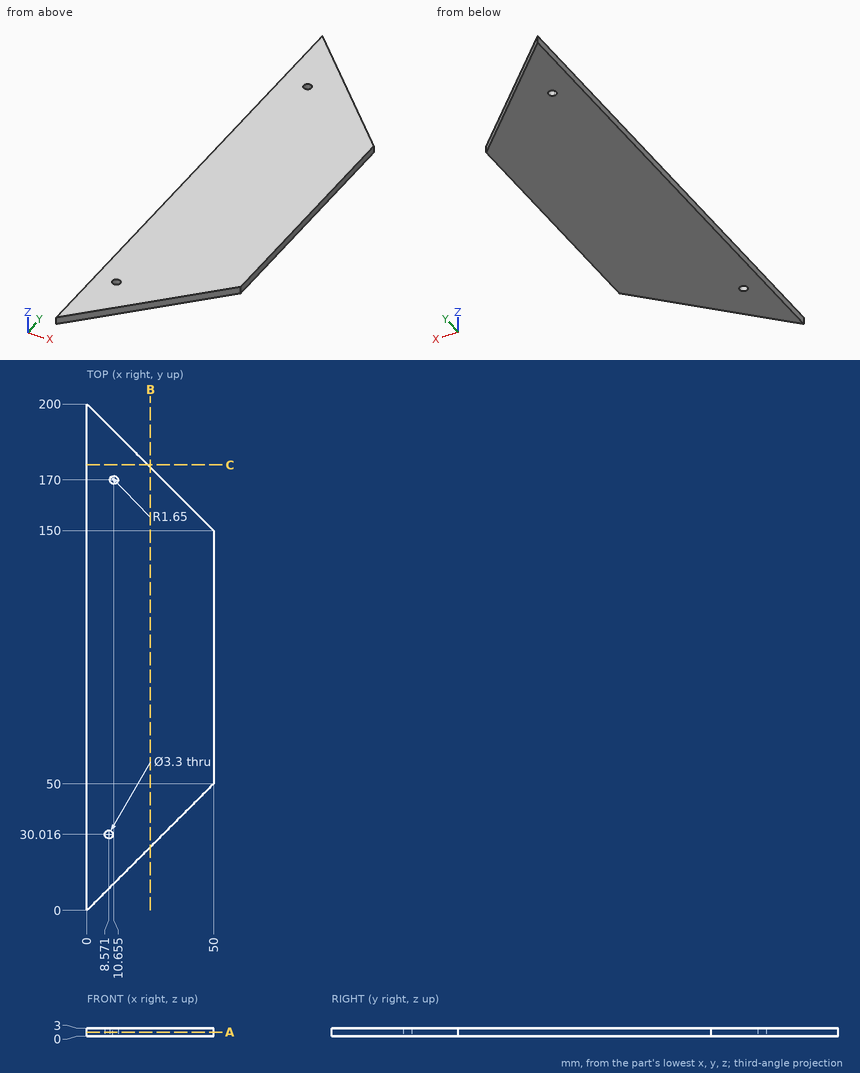
Geometry check sheet. Reference: drawing and pictorial views, mm from the part's lowest x, y, z. Round coordinates to 2 decimals unless told otherwise and drop trailing zeros. Loops run counter-clockwise (first coordinate to the right, second up) from the corner with the lowest first, then second, coordinate; pieces in that order, holes last. Notation, with made-up numbers: (54, -22) - (89, -22) arc R23 cw to (89, -6) - close; hole circle Ø7 at (14.25, -22.5). An arc over 180 degrees is marked (long way). Answer in a Markdown table with one row per item. Add a question column.
Q1. Section check C-C on y = 176. Enter the section's corners in (x, z).
Q2. Section check B-B on x = 25. Enter the section's corners in (y, z), plus the area to 3 significant figures.
Q3. Gauge pin test, flat end, axial feed: pin 1 (3 mm diameter, centred on x = 32, y = 40, fed in from -Z). Record the tip position at first contact, or that the pin passes through.
Q4. Section check A-A on z = 1.55. State how many separate pieces and enclosed holes the cut face has, plus the area to 3 significant figures.
Q5. Material ranges on line 1 (Y direction, x = 10, z = 2.35) (1 decimal); line 2 (Y direction, x = 36, z = 1.35); line 3 (Y direction, x = 30.5, z = 0.5), recorded low to high.
Found:
| question | item | result |
|---|---|---|
| 1 | outline | (0, 0) - (24, 0) - (24, 3) - (0, 3) - close |
| 2 | outline | (25, 0) - (175, 0) - (175, 3) - (25, 3) - close |
| 2 | area | 450 mm² |
| 3 | pin 1 | stops at z = 0 |
| 4 | separate pieces | 1 |
| 4 | enclosed holes | 2 |
| 4 | area | 7,480 mm² |
| 5 | line 1 | y = 10 to 29.2, 30.8 to 168.5, 171.5 to 190 |
| 5 | line 2 | y = 36 to 164 |
| 5 | line 3 | y = 30.5 to 169.5 |
